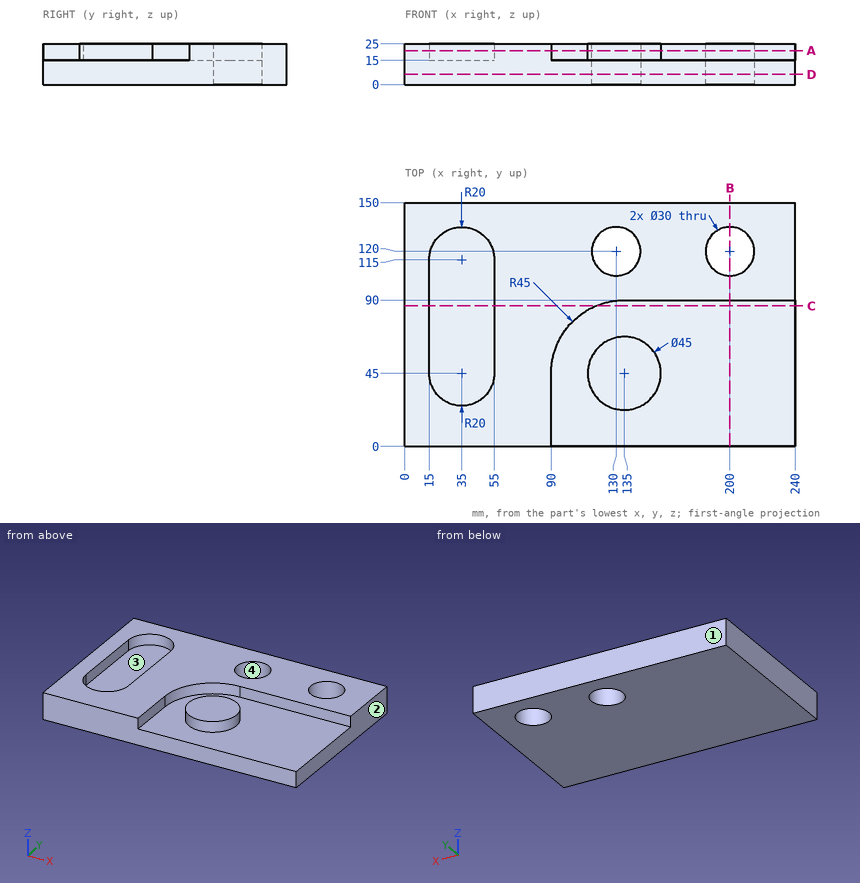
For this review, use the dimensioned drawing (mm, ordinates from the lowest corner) and the shaded views. Round coordinates to 2 decimals unless told otherwise and drop trailing zeros. Write each loop counter-clockwise with the first axis right and the second up, starting at its lowest first coordinate (ties: lowest second). Pieces come first, ordered by that corner, then holes. Notation, with made-up numbers: (8, -10.75) - (25, -10.75) arc R21 cw to (25, 4.25) - close; hole circle Ø7 at (45, 76). An arc over 180 degrees is marked (long way). Use CSV: the item, a comma, the result in double quotes.
1) Add section C-C on y = 86.5. Write out the cut boundary in (x, z), and give its area (3 significant figures).
Conclusion:
outline,"(0, 0) - (240, 0) - (240, 15) - (117.6, 15) - (117.6, 25) - (55, 25) - (55, 15) - (15, 15) - (15, 25) - (0, 25) - close"
area,"4,380 mm^2"
2) Add section D-D on z = 6.25. Write out the cut boundary in (x, y).
Conclusion:
outline,"(0, 0) - (240, 0) - (240, 150) - (0, 150) - close; hole circle Ø30 at (130, 120); hole circle Ø30 at (200, 120)"
3) Add section B-B on x = 200. Write out the cut boundary in (y, z), and give its area (3 significant figures).
Conclusion:
outline,"(0, 0) - (105, 0) - (105, 25) - (90, 25) - (90, 15) - (0, 15) - close; (135, 0) - (150, 0) - (150, 25) - (135, 25) - close"
area,"2,100 mm^2"
4) Clearance check with flat-ended pins moving along their axes: pin 1 Ø3 at (y, z) = (72.5, 19.5) entering from +X; pin 2 Ø12 at (x, y) = (40.5, 60) entering from +Z; pin 3 Ø3 at (x, z) = (208.5, 19.5) entering from -Y. State where each tip first meets the part, or that it passes through.
Conclusion:
pin 1,"stops at x = 100.59"
pin 2,"stops at z = 15"
pin 3,"stops at y = 90"
5) Wall thickness on line 1 along X through (y, z) = (119.5, 5); line 2 along Y through (x, z) = (130, 7); line 3 along X through (y, z) = (115, 6.5): over which ranges is each line inside the solid? List them lowest first. Write a range as from..to.
Conclusion:
line 1,"x = 0..115.01, 144.99..185.01, 214.99..240"
line 2,"y = 0..105, 135..150"
line 3,"x = 0..115.86, 144.14..185.86, 214.14..240"
6) The part is to be moulded in two halves that separate along Y. For the marked faces 1, 2, 3 and 4, say which applies: pulls with the +Y half, pulls with the -Y half, needs draft (parallel to the pull), parting line crosses it, or undercut.
Conclusion:
face 1,"pulls with the +Y half"
face 2,"needs draft"
face 3,"undercut"
face 4,"undercut"
7) Add section A-A on z = 21. Write out the cut boundary in (x, y), and give its area (3 significant figures).
Conclusion:
outline,"(0, 0) - (90, 0) - (90, 45) arc R45 cw to (135, 90) - (240, 90) - (240, 150) - (0, 150) - close; circle Ø45 at (135, 45); hole (15, 45) arc R20 ccw to (55, 45) - (55, 115) arc R20 ccw to (15, 115) - close; hole circle Ø30 at (130, 120); hole circle Ø30 at (200, 120)"
area,"19,100 mm^2"
